```python
from build123d import *

# Parameters (mm, degrees)
F0_W     = 550
F0_H     = 80
F0_W_2   = 69
F0_H_2   = 41
F0_R     = 14
F1_DEPTH = 10
F2_R     = 4


with BuildPart() as f1:
    # F0 (on Front) → F1 (new body)
    with BuildSketch(Plane.XZ):
        Rectangle(F0_W, F0_H)
        with Locations((0, -4.5)):
            Rectangle(F0_W_2, F0_H_2, mode=Mode.SUBTRACT)
        with Locations((-167.5, 0)):
            Circle(F0_R, mode=Mode.SUBTRACT)
        with Locations((-107.5, 0)):
            Circle(F0_R, mode=Mode.SUBTRACT)
        with Locations((107.5, 0)):
            Circle(F0_R, mode=Mode.SUBTRACT)
        with Locations((167.5, 0)):
            Circle(F0_R, mode=Mode.SUBTRACT)
    extrude(amount=-F1_DEPTH)

    # F2
    f2_edges = [f1.edges().sort_by_distance(p)[0] for p in [
        (-34.5, 5, 16),
        (34.5, 5, 16),
        (34.5, 5, -25),
        (-34.5, 5, -25),
    ]]
    fillet(f2_edges, radius=F2_R)


solid = f1.part
```
Verification items for the finished model (mm, model axes). A direction names the side the tool comes from. Give positions to 0.01 mm unless a question says otherwise; leave off trailing zeros. Write each loop counter-clockwise with the first axis right and the second up, starting at its lowest first coordinate (ties: lowest second). Pieces come first, ordered by that corner, then holes. Notation, with made-up numbers: (-19, 67.25) - (0, 67.25) arc R16 ccw to (0, 81.25) - close; hole circle Ø4 at (-30, -34.5). An arc over 180 degrees is marked (long way). Put each result on its own line as item: value.
Q1. Section check C-C on y = 3.25. Record the cut outline in (x, z), and give its area (3 significant figures).
Result:
outline: (-275, -40) - (275, -40) - (275, 40) - (-275, 40) - close; hole circle Ø28 at (-167.5, 0); hole circle Ø28 at (-107.5, 0); hole (-34.5, -21) arc R4 ccw to (-30.5, -25) - (30.5, -25) arc R4 ccw to (34.5, -21) - (34.5, 12) arc R4 ccw to (30.5, 16) - (-30.5, 16) arc R4 ccw to (-34.5, 12) - close; hole circle Ø28 at (107.5, 0); hole circle Ø28 at (167.5, 0)
area: 38,700 mm2
Q2. Scan lines: probe 1 along X at (y, z) = (5, -1); probe 2 along Z at (x, y) = (167.5, 7.5); probe 3 along Z at (x, y) = (169, 1.5). Record each from-to range of solid material in increasing order. Write a range as from..to.
Result:
probe 1: -275..-181.46, -153.54..-121.46, -93.54..-34.5, 34.5..93.54, 121.46..153.54, 181.46..275
probe 2: -40..-14, 14..40
probe 3: -40..-13.92, 13.92..40
Q3. Set-up check for faces 4 (the face through (275, 5, -1)), 5 (the face through (34.5, 5, -5)): record each of +Z, -Z, +X, -X, +Y, -Y from which the full face is reachable in a straight line by a thin tool's end or side.
Result:
face 4: +Z, -Z, +X, +Y, -Y
face 5: +Y, -Y
Q4. Mould release check, pull along Z, two halves, no side actions. Record for faces 1 (the face through (-275, 5, -1)), 2 (the face through (-181.486, 4.93, 0.616)), 3 (the face through (-4, 5, -40)): released by +Z, released by -Z, zero draft, split by the parting line, or undercut.
Result:
face 1: zero draft
face 2: undercut
face 3: released by -Z
Q5. Section check A-A on x = -107.5. Record the cut outline in (y, z).
Result:
outline: (0, -40) - (10, -40) - (10, -14) - (0, -14) - close; (0, 14) - (10, 14) - (10, 40) - (0, 40) - close
Q6. Section check B-B on z = 0. Record the cut outline in (x, y).
Result:
outline: (-275, 0) - (-181.5, 0) - (-181.5, 10) - (-275, 10) - close; (-153.5, 0) - (-121.5, 0) - (-121.5, 10) - (-153.5, 10) - close; (-93.5, 0) - (-34.5, 0) - (-34.5, 10) - (-93.5, 10) - close; (34.5, 0) - (93.5, 0) - (93.5, 10) - (34.5, 10) - close; (121.5, 0) - (153.5, 0) - (153.5, 10) - (121.5, 10) - close; (181.5, 0) - (275, 0) - (275, 10) - (181.5, 10) - close
